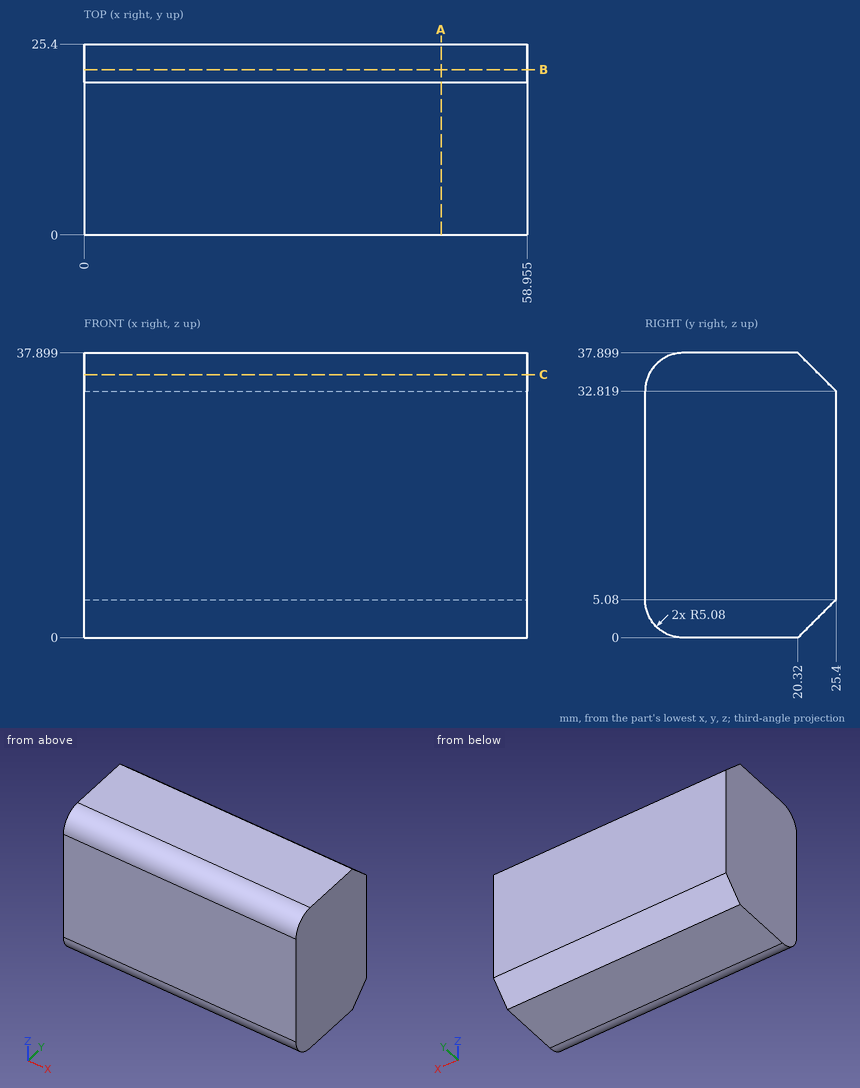
Print and shaded views of the part. All mm, measured from the part's lowest x, y and z. Coordinates: 2 decimals unless noted, no trailing zeros. Order: outer loops, then holes, each group sorted by start corner. A loop starts at its lowest first (then second) coordinate and runs counter-clockwise, first axis right, second up. Notation, with made-up numbers: M 45,70.25 L 99,70.25 A17 cw 99,101.25 Z; hole C 42,34 d6. An arc over 180 degrees is marked long. Answer as CSV lines item,"result".
1) Cut at B-B (y = 22). List the corners of the cut face in (x, z) (1 decimal), then the cut area to 3 significant figures.
Verdict:
outline,"M 0,1.7 L 59,1.7 L 59,36.2 L 0,36.2 Z"
area,"2,040 mm2"
2) Cut at A-A (x = 47.5). List the corners of the cut face in (y, z).
Verdict:
outline,"M 0,5.08 A5.08 ccw 5.08,0 L 20.32,0 L 25.4,5.08 L 25.4,32.82 L 20.32,37.9 L 5.08,37.9 A5.08 ccw 0,32.82 Z"
3) Drill centre lines: L1, parallel to Z at x = 41.5, y = 5; L2, parallel to Y at x = 46, z = 35.5 (1 decimal); L3, parallel to Y at x = 19, z = 35. Where is each one in solid material? Low to high. Write a range as from..to.
Verdict:
L1,"0..37.9"
L2,"0.8..22.7"
L3,"0.49..23.22"
4) Cut at C-C (z = 35). List the corners of the cut face in (x, y) (1 decimal).
Verdict:
outline,"M 0,0.5 L 59,0.5 L 59,23.2 L 0,23.2 Z"
